Geometry: final body of the model. Coordinates: model frame, mm. A direction names the side the tool comes from. Round coordinates to 2 decimals unless told otherwise and drop trailing zeros. Loops run counter-clockwise (first coordinate to the right, second up) from the corner with the lowest first, then second, coordinate; pieces in that order, holes last. Notation, with made-up numbers: M 78.25,83 L 135.25,83 A25 ccw 135.25,106 Z; hole C 15.25,85 d10. An arc over 180 degrees is marked long. Answer as a JSON object with one key per item and string values.
from build123d import *

# Parameters (mm, degrees)
BOSS_EXTRUDE1_DEPTH = 6.4
SKETCH3_R           = 1.1
CUT_EXTRUDE1_DEPTH  = 14.148478999
BOSS_EXTRUDE2_START = 0.15
SKETCH4_R           = 1.1
BOSS_EXTRUDE2_DEPTH = 6.7
SKETCH5_W           = 0.5
SKETCH5_H           = 3.35
BOSS_EXTRUDE3_DEPTH = 4.4
SKETCH6_W           = 0.5
SKETCH6_H           = 3.35
BOSS_EXTRUDE4_DEPTH = 4.4
EXTRUDE_THIN2_START = -1
EXTRUDE_THIN2_DEPTH = 4


with BuildPart() as part:
    # Sketch1 → Boss-Extrude1 (new body)
    with BuildSketch(Plane.XY):
        Polygon((-10, 4.85), (0, 4.85), (0.64599961, 5.65), (10, 5.65), (10, 4.85), (10, -4.85), (-10, -4.85), align=None)
    extrude(amount=BOSS_EXTRUDE1_DEPTH)

    # Sketch3 → Cut-Extrude1 (cut, through all)
    with BuildSketch(Plane.XY.offset(6.4)):
        with Locations((-4.9, -2.45)):
            Circle(SKETCH3_R)
    cut_extrude1 = extrude(amount=-CUT_EXTRUDE1_DEPTH, mode=Mode.SUBTRACT)

    # Sketch4 → Boss-Extrude2 (add)
    with BuildSketch(Plane.XY.offset(6.4).offset(BOSS_EXTRUDE2_START)):
        with BuildLine():
            Line((-6.55, -2.45), (-6.55, -5.25))
            Line((-6.55, -5.25), (-3.25, -5.25))
            Line((-3.25, -5.25), (-3.25, -2.45))
            ThreePointArc((-3.25, -2.45), (-4.9, -0.8), (-6.55, -2.45))
        make_face()
        with Locations((-4.9, -2.45)):
            Circle(SKETCH4_R, mode=Mode.SUBTRACT)
    boss_extrude2 = extrude(amount=-BOSS_EXTRUDE2_DEPTH)

    # Sketch5 → Boss-Extrude3 (add)
    with BuildSketch(Plane.XZ.offset(4.85)):
        with Locations((-7.85, 3.425)):
            Rectangle(SKETCH5_W, SKETCH5_H)
    boss_extrude3 = extrude(amount=BOSS_EXTRUDE3_DEPTH)

    # Sketch6 → Boss-Extrude4 (add)
    with BuildSketch(Plane(origin=(0, -4.85, -4.85), x_dir=(-1, 0, 0), z_dir=(0, 1, 0))):
        with Locations((0, 8.275)):
            Rectangle(SKETCH6_W, SKETCH6_H)
    extrude(amount=-BOSS_EXTRUDE4_DEPTH)

    # Mirror1: Cut-Extrude1, Boss-Extrude2, Boss-Extrude3 across plane
    add(cut_extrude1.mirror(Plane(origin=(0, 0, 0), x_dir=(0, 0, 1), z_dir=(1, 0, 0))), mode=Mode.SUBTRACT)
    add(boss_extrude2.mirror(Plane(origin=(0, 0, 0), x_dir=(0, 0, 1), z_dir=(1, 0, 0))))
    add(boss_extrude3.mirror(Plane(origin=(0, 0, 0), x_dir=(0, 0, 1), z_dir=(1, 0, 0))))

    # Sketch7 → Extrude-Thin2 (add)
    with BuildSketch(Plane(origin=(0, 0, 0), x_dir=(-1, 0, 0), z_dir=(0, 0, -1)).offset(EXTRUDE_THIN2_START)):
        with BuildLine():
            Line((-7.1, 5.65), (-7.1, 6.15))
            ThreePointArc((-7.1, 6.15), (-6.986771965, 6.466871341), (-6.698370212, 6.640227806))
            Line((-6.698370212, 6.640227806), (8.55, 9.7))
            Line((8.55, 9.7), (8.609022127, 9.405863317))
            Line((8.609022127, 9.405863317), (-6.639348085, 6.346091122))
            ThreePointArc((-6.639348085, 6.346091122), (-6.754708786, 6.276748537), (-6.8, 6.15))
            Line((-6.8, 6.15), (-6.8, 5.65))
            Line((-6.8, 5.65), (-7.1, 5.65))
        make_face()
    extrude(amount=-EXTRUDE_THIN2_DEPTH)


solid = part.part
1) Section query B-B (z = 1.5). Return the cut outline in (x, y).
Results:
{"outline": "M -10,-4.85 L -6.55,-4.85 L -6.55,-5.25 L -3.25,-5.25 L -3.25,-4.85 L 3.25,-4.85 L 3.25,-5.25 L 6.55,-5.25 L 6.55,-4.85 L 10,-4.85 L 10,5.65 L 7.1,5.65 L 7.1,6.15 A0.5 ccw 6.7,6.64 L -8.55,9.7 L -8.61,9.41 L 6.64,6.35 A0.2 cw 6.8,6.15 L 6.8,5.65 L 0.65,5.65 L 0,4.85 L -10,4.85 Z; hole C -4.9,-2.45 d2.2; hole C 4.9,-2.45 d2.2"}
2) Pin query (flat end, axial travel): P1, Ø3.5, axis at y = -7, z = 3.5, coming from the +X side; P2, Ø1, axis at x = -4.5, z = 4, coming from the -Y side; P3, Ø4, axis at x = 4.5, y = 7, coming from the -Z side; P4, Ø2.5, axis at y = -6, z = 3.5, coming from the -X side. Return the tip coordinate at first contact, or that it passes through.
Results:
{"P1": "x = 8.1", "P2": "y = -5.25", "P3": "z = 0", "P4": "x = -10"}
3) Pull-direction query (Y, two-part tool) for faces 1 (the cylindrical face through (3.85, -2.12, 3.25)), 2 (the flat face through (5, -5.25, 3)), 3 (the flat face through (-3.25, -5, 3)); classes: +Y half, -Y half, draft (parallel to the pull), parting line (faces both ways), or undercut.
Results:
{"face 1": "undercut", "face 2": "-Y half", "face 3": "draft"}
4) Reachability of faces 4 (the flat face through (8.1, -7, 3)), 5 (the flat face through (-10, 0, 3)), 6 (the flat face through (-8.1, -7, 3)), 7 (the flat face through (0.25, -7, 3)), 8 (the flat face through (0.318, 5.244, 3.155)) from +Z, -Z, +X, -X, +Y, -Y: full face, straight path, thin tool, end or side. Return the list, or none.
Results:
{"face 4": "+Z, -Z, +X, -Y", "face 5": "+Z, -Z, -X, +Y, -Y", "face 6": "+Z, -Z, -X, -Y", "face 7": "+Z, -Z, -Y", "face 8": "+Z, -Z, -X"}
5) Section query A-A (x = 4.9). Return the cut outline in (y, z).
Results:
{"outline": "M -5.25,-0.15 L -3.55,-0.15 L -3.55,6.55 L -5.25,6.55 Z; M -1.35,-0.15 L -0.8,-0.15 L -0.8,0 L 5.65,0 L 5.65,6.4 L -0.8,6.4 L -0.8,6.55 L -1.35,6.55 Z; M 6.7,1 L 7,1 L 7,5 L 6.7,5 Z"}
6) Section query C-C (y = -1.75). Return the cut outline in (x, z).
Results:
{"outline": "M -10,0 L -6.39,0 L -6.39,-0.15 L -5.75,-0.15 L -5.75,6.55 L -6.39,6.55 L -6.39,6.4 L -10,6.4 Z; M -4.05,-0.15 L -3.41,-0.15 L -3.41,0 L 3.41,0 L 3.41,-0.15 L 4.05,-0.15 L 4.05,6.55 L 3.41,6.55 L 3.41,6.4 L -3.41,6.4 L -3.41,6.55 L -4.05,6.55 Z; M 5.75,-0.15 L 6.39,-0.15 L 6.39,0 L 10,0 L 10,6.4 L 6.39,6.4 L 6.39,6.55 L 5.75,6.55 Z"}
7) Section query D-D (x = 2.75). Return the cut outline in (y, z), and give its area (3 significant figures).
Results:
{"outline": "M -4.85,0 L 5.65,0 L 5.65,6.4 L -4.85,6.4 Z; M 7.13,1 L 7.43,1 L 7.43,5 L 7.13,5 Z", "area": "68.4 mm2"}
8) Ray query, line 1 (Y direction, x = -4.9, z = 5.25); line 2 (Y direction, x = -4.9, z = 2.5); line 3 (Y direction, x = 5.5, z = 1.75). Return the intervals inside material, ascending.
Results:
{"line 1": "-5.25 to -3.55, -1.35 to 4.85", "line 2": "-5.25 to -3.55, -1.35 to 4.85, 8.66 to 8.97", "line 3": "-5.25 to -3.37, -1.53 to 5.65, 6.57 to 6.88"}
